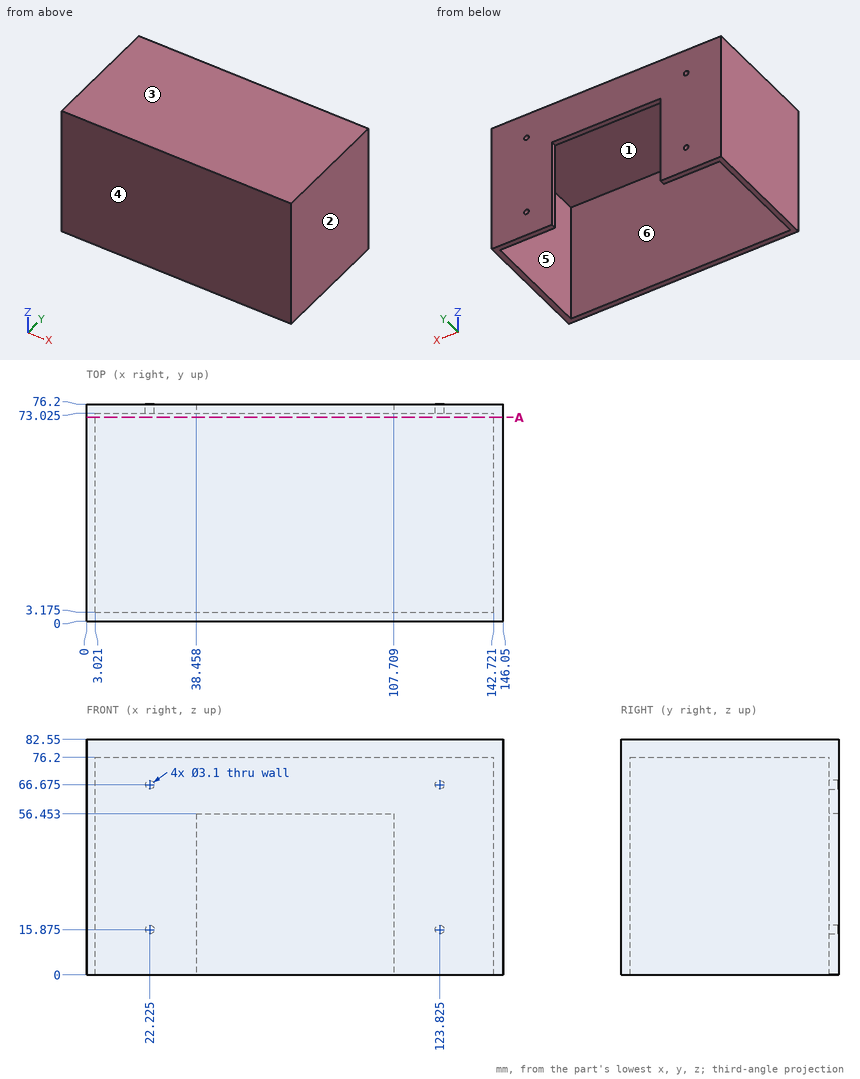
Could you check a few things on this drawing? It's one solid part, dimensions in mm from its lowest x, y, z. A direction names the side the tool comes from. Round coordinates to 2 decimals unless told otherwise and drop trailing zeros. Order: outer loops, then holes, each group sorted by start corner. A loop starts at its lowest first (then second) coordinate and runs counter-clockwise, first axis right, second up.
Q1. Please list where these lines run through material, in increasing order: probe 1 along Y at (x, z) = (79.5, 62) (1 decimal); probe 2 along X at (y, z) = (54, 16.5); probe 3 along Z at (x, y) = (128, 71.5).
Geometry says:
probe 1: y = 0 to 3.2, 73 to 76.2
probe 2: x = 0 to 3.02, 142.72 to 146.05
probe 3: z = 76.2 to 82.55
Q2. Thinking about a two-plate mould opening in Y: for the marked faces 3, 4, 5 and 6, which applies, released by +Y, released by -Y, zero draft, split by the parting line, or undercut?
Geometry says:
face 3: zero draft
face 4: released by -Y
face 5: undercut
face 6: undercut
Q3. I'm going to push flat-ended pins straight in: P1, Ø3, axis at x = 77.5, z = 44.5, coming from the +Y side (3 decimals); P2, Ø1, axis at y = 75, z = 42, coming from the -X side; P3, Ø2.5, axis at x = 79.5, y = 75, coming from the -Z side. Where does each tip first touch, or does it pass through?
Geometry says:
P1: stops at y = 3.175
P2: stops at x = 0
P3: stops at z = 56.45
Q4. Which directions (+Z, -Z, +X, -X, +Y, -Y) give clear straight access to the entire face, cutting with the end or side of a thin tool? Please do the marked faces 1 and 2.
Geometry says:
face 1: -Z
face 2: +Z, -Z, +X, +Y, -Y
Q5. Imagine slicing it at A-A, the plane y = 71.5. List the corners of the cut face in (x, z) for me.
Geometry says:
outline: (0, 0) - (3.02, 0) - (3.02, 76.2) - (142.72, 76.2) - (142.72, 0) - (146.05, 0) - (146.05, 82.55) - (0, 82.55) - close
